The drawing under review shows one solid part. Ordinate dimensions are in mm from its lowest x, y, z. Coordinates: 2 decimals unless noted, no trailing zeros. Order: outer loops, then holes, each group sorted by start corner. A loop starts at its lowest first (then second) coordinate and runs counter-clockwise, first axis right, second up. Notation, with made-up numbers: (53.5, 59) -> (76.5, 59) arc R37 ccw to (76.5, 98) -> close; hole circle Ø9 at (-17, 82.5). An arc over 180 degrees is marked (long way). Write item = value, one per line.
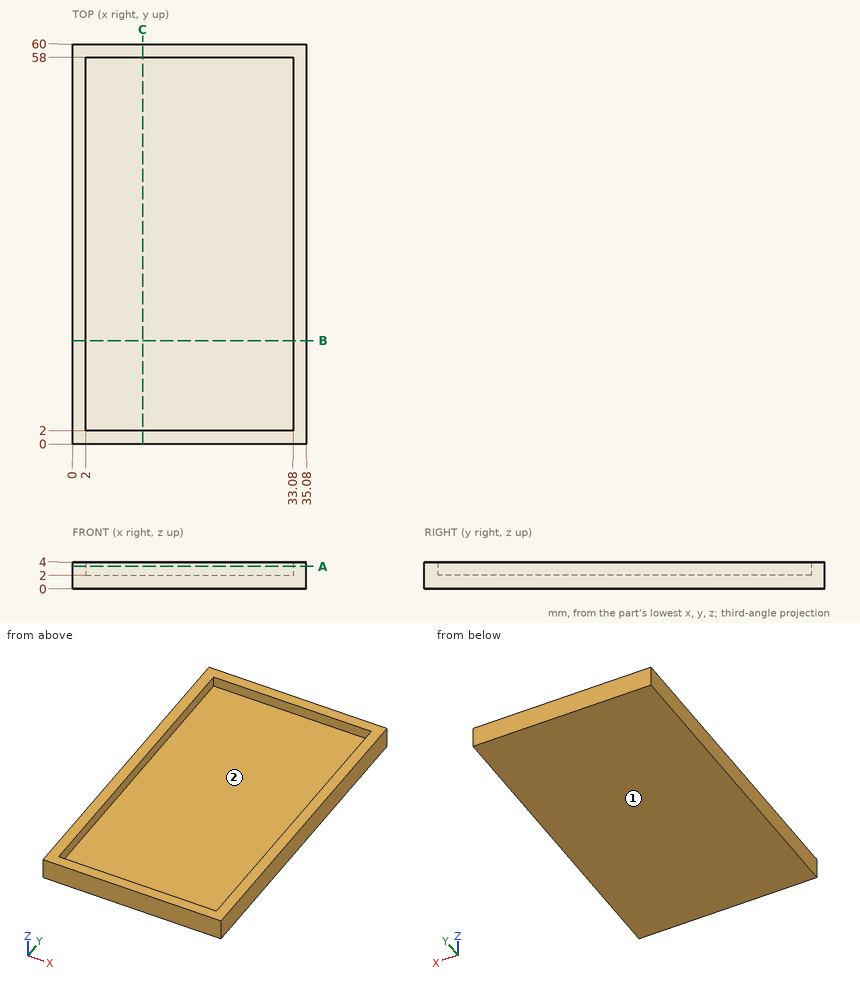
(1) For L1, parallel to X at y = 19.5, z = 2.5; L2, parallel to Y at x = 23, z = 2.15; L3, parallel to Z at x = 29, y = 57.5, list the stretches that pass through material, from the lowest coordinate up.
Report:
L1 = 0 to 2, 33.08 to 35.08
L2 = 0 to 2, 58 to 60
L3 = 0 to 2
(2) Insertion check: pin 1 (12 mm diameter, centred on x = 21, y = 41.5, fed in from +Z). The pin has a flat end and moves straight along its axis. Give the tip position at first contact, or say it passes through.
Report:
pin_1 = 2
(3) We need section C-C (x = 10.5). Write out the cut boundary in (y, z), and give its area (3 significant figures).
Report:
outline = (0, 0) -> (60, 0) -> (60, 4) -> (58, 4) -> (58, 2) -> (2, 2) -> (2, 4) -> (0, 4) -> close
area = 128 mm²
(4) We need section A-A (z = 3.35). Write out the cut boundary in (x, y), and give its area (3 significant figures).
Report:
outline = (0, 0) -> (35.08, 0) -> (35.08, 60) -> (0, 60) -> close; hole (2, 2) -> (33.08, 2) -> (33.08, 58) -> (2, 58) -> close
area = 364 mm²
(5) We need section B-B (y = 15.5). Write out the cut boundary in (x, z).
Report:
outline = (0, 0) -> (35.08, 0) -> (35.08, 4) -> (33.08, 4) -> (33.08, 2) -> (2, 2) -> (2, 4) -> (0, 4) -> close
(6) The part is to be moulded in two halves that separate along X. For the marked faces 1 and 2, say which applies: released by +X, released by -X, zero draft, split by the parting line, or undercut.
Report:
face_1 = zero draft
face_2 = undercut
